from build123d import *

# Parameters (mm, degrees)
F0_W     = 38.1
F0_H     = 38.1
F1_DEPTH = 50.8
F2_R     = 12.7
F3_DEPTH = 50.801


with BuildPart() as f1:
    # F0 (on Top) → F1 (new body)
    with BuildSketch(Plane.XY):
        with BuildLine():
            ThreePointArc((0, 6.35), (1.859872, 1.859872), (6.35, 0))
            Line((6.35, 0), (44.45, 0))
            ThreePointArc((44.45, 0), (48.940128, 1.859872), (50.8, 6.35))
            Line((50.8, 6.35), (50.8, 44.45))
            ThreePointArc((50.8, 44.45), (48.940128, 48.940128), (44.45, 50.8))
            Line((44.45, 50.8), (6.35, 50.8))
            ThreePointArc((6.35, 50.8), (1.859872, 48.940128), (0, 44.45))
            Line((0, 44.45), (0, 6.35))
        make_face()
        with Locations((25.4, 25.4)):
            Rectangle(F0_W, F0_H, mode=Mode.SUBTRACT)
    extrude(amount=F1_DEPTH)

    # F2 (on face) → F3 (cut, through all)
    with BuildSketch(Plane.XZ):
        with Locations((25.4, 25.4)):
            Circle(F2_R)
    extrude(amount=-F3_DEPTH, mode=Mode.SUBTRACT)


solid = f1.part
Could you check a few things on this model? Use its own coordinates, in mm. A direction names the side the tool comes from. Round coordinates to 2 decimals unless told otherwise and drop trailing zeros. Write each loop counter-clockwise with the first axis right and the second up, starting at its lowest first coordinate (ties: lowest second). Pieces come first, ordered by that corner, then holes. Notation, with made-up numbers: (69, 18.5) - (92, 18.5) arc R13 ccw to (92, 43.5) - close; hole circle Ø5 at (79, -25.5). An arc over 180 degrees is marked (long way). Put each result on its own line as item: value. Start each with the question number.
(1) I want a section at A-A, the plane y = 37. Please give me the cut outline in (x, z), plus the area to 3 significant figures.
(2) For faces 4 (the flat face through (38.4, 50.8, 25)), 5 (the flat face through (44.45, 25, 25)), which set-ups out of +Z, -Z, +X, -X, +Y, -Y let a thin tool reach every point of the face, with its end or its side?
(3) I need wall thicknesses on probe 1 along X at (y, z) = (44, 39.5); probe 2 along Z at (x, y) = (25.4, 4). Which ranges of each line are inside material? Lowest first, please.
(4) Thinking about a two-plate mould opening in X: for faces 1 (the cylindrical face through (16.04, 47.581, 33.983)), 2 (the flat face through (48, 26, 0)), 3 (the cylindrical face through (1.91, 48.99, 25.04)), which applies, released by +X, released by -X, zero draft, split by the parting line, or undercut?
(5) I want a section at B-B, the plane z = 5. Please give me the cut outline in (x, y).
(6) I want a section at D-D, the plane z = 25.4. Please give me the cut outline in (x, y), plus the area to 3 significant figures.
(7) Will this pin go through, and if not, where does the flat tip stop? pin 1 (6 mm diameter, centred on x = 15, y = 41.5, fed in from -Z).
Here are the results:
1. outline: (0, 0) - (6.35, 0) - (6.35, 50.8) - (0, 50.8) - close; (44.45, 0) - (50.8, 0) - (50.8, 50.8) - (44.45, 50.8) - close
1. area: 645 mm^2
2. face 4: +Z, -Z, +X, -X, +Y
2. face 5: +Z, -Z
3. probe 1: x = 0 to 6.35, 44.45 to 50.8
3. probe 2: z = 0 to 12.7, 38.1 to 50.8
4. face 1: undercut
4. face 2: zero draft
4. face 3: released by -X
5. outline: (0, 6.35) arc R6.35 ccw to (6.35, 0) - (44.45, 0) arc R6.35 ccw to (50.8, 6.35) - (50.8, 44.45) arc R6.35 ccw to (44.45, 50.8) - (6.35, 50.8) arc R6.35 ccw to (0, 44.45) - close; hole (6.35, 6.35) - (44.45, 6.35) - (44.45, 44.45) - (6.35, 44.45) - close
6. outline: (0, 6.35) arc R6.35 ccw to (6.35, 0) - (12.7, 0) - (12.7, 6.35) - (6.35, 6.35) - (6.35, 44.45) - (12.7, 44.45) - (12.7, 50.8) - (6.35, 50.8) arc R6.35 ccw to (0, 44.45) - close; (38.1, 0) - (44.45, 0) arc R6.35 ccw to (50.8, 6.35) - (50.8, 44.45) arc R6.35 ccw to (44.45, 50.8) - (38.1, 50.8) - (38.1, 44.45) - (44.45, 44.45) - (44.45, 6.35) - (38.1, 6.35) - close
6. area: 772 mm^2
7. pin 1: stops at z = 0
